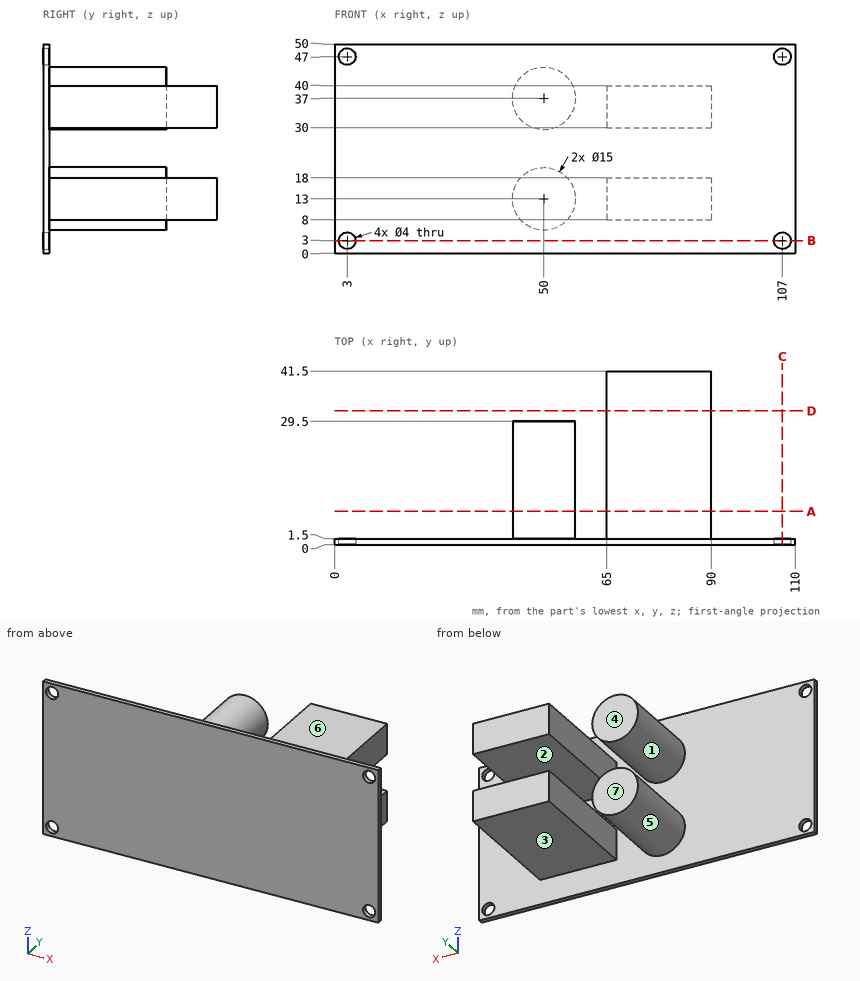
Could you check a few things on this drawing? It's one solid part, dimensions in mm from its lowest x, y, z. A direction names the side the tool comes from. Coordinates: 2 decimals unless noted, no trailing zeros. Order: outer loops, then holes, each group sorted by start corner. A loop starts at its lowest first (then second) coordinate and runs counter-clockwise, first axis right, second up. Notation, with made-up numbers: M -35.5,12.25 L 20.5,12.25 A14 cw 20.5,16.25 Z; hole C 75,-8.5 d11. An arc over 180 degrees is marked long. Use a Markdown table: item, result. Add a question column.
Q1. I want a section at B-B on z = 3. List the corners of the cut face in (x, y) for me, then the cut area to 3 significant figures.
Q2. I'm going to push flat-ended pins straight in: pin 1 (2 mm diameter, centred on x = 76.5, y = 23, fed in from -Z); pin 2 (10 mm diameter, centred on y = 35, z = 8.5, fed in from +X); pin 3 (3 mm diameter, centred on x = 3, z = 3, fed in from -Y); pin 4 (7.5 mm diameter, centred on x = 47.5, z = 37.5, fed in from +Y). Where does each tip first touch, or does it pass through?
Q3. We'd pull the mould along Z, two halves only. Please class the marked faces 1, 2, 3 and 4: pulls with the +Z half, pulls with the -Z half, needs draft (parallel to the pull), parting line crosses it, or undercut.
Q4. I want a section at A-A on y = 8. List the corners of the cut face in (x, z) for me.
Q5. I want a section at C-C on x = 107. List the corners of the cut face in (y, z) for me, then the cut area to 3 significant figures.
Q6. I want a section at D-D on y = 32. List the corners of the cut face in (x, z) for me.
Q7. Which directions (+Z, -Z, +X, -X, +Y, -Y) give clear straight access to the entire face, cutting with the end or side of a thin tool? Please do the marked faces 5, 6 and 7.
Q8. If I drill on L1, parallel to X at y = 0.95, z = 47; L2, parallel to Z at x = 107, y = 0.8; L3, parallel to Z at x = 78, y = 39.5, over which ranges is the centre line in solid material (lowest first)?
Checked values:
| question | item | result |
|---|---|---|
| 1 | outline | M 0,0 L 1,0 L 1,1.5 L 0,1.5 Z; M 5,0 L 105,0 L 105,1.5 L 5,1.5 Z; M 109,0 L 110,0 L 110,1.5 L 109,1.5 Z |
| 1 | area | 153 mm² |
| 2 | pin 1 | z = 8 |
| 2 | pin 2 | x = 90 |
| 2 | pin 3 | through |
| 2 | pin 4 | y = 29.5 |
| 3 | face 1 | undercut |
| 3 | face 2 | undercut |
| 3 | face 3 | pulls with the -Z half |
| 3 | face 4 | needs draft |
| 4 | outline | C 50,13 d15; C 50,37 d15; M 65,8 L 90,8 L 90,18 L 65,18 Z; M 65,30 L 90,30 L 90,40 L 65,40 Z |
| 5 | outline | M 0,0 L 1.5,0 L 1.5,1 L 0,1 Z; M 0,5 L 1.5,5 L 1.5,45 L 0,45 Z; M 0,49 L 1.5,49 L 1.5,50 L 0,50 Z |
| 5 | area | 63.0 mm² |
| 6 | outline | M 65,8 L 90,8 L 90,18 L 65,18 Z; M 65,30 L 90,30 L 90,40 L 65,40 Z |
| 7 | face 5 | +Y |
| 7 | face 6 | +Z, +X, +Y |
| 7 | face 7 | +Z, -Z, -X, +Y |
| 8 | L1 | 0 to 1, 5 to 105, 109 to 110 |
| 8 | L2 | 0 to 1, 5 to 45, 49 to 50 |
| 8 | L3 | 8 to 18, 30 to 40 |
